Autodesk Fusion 360 part; units mm, degrees
sketch "top view" plane through (0, 0, 0) normal (0, 0, 1) x (1, 0, 0)
  line L0 (12.0004, 0) -> (29.9996, 0)
  line L1 (42, 12) -> (42, 66)
  line L2 (42, 66) -> (0, 66)
  line L3 (0, 66) -> (0, 0) construction
  line L4 (21, 66) -> (21, 0) construction
  line L5 (0, 66) -> (15, 66)
  line L6 (15, 54) -> (15, 0)
  line L7 (15, 0) -> (12.0004, 0) construction
  line L8 (0, 12) -> (0, 66)
  line L9 (27, 54) -> (27, 0)
  line L10 (0, 0) -> (12.0004, 0) construction
  line L11 (12.0004, 0) -> (12.0004, 12) construction
  line L12 (12.0004, 12) -> (0, 12) construction
  line L13 (0, 12) -> (0, 0) construction
  line L14 (0, 12) -> (12.0004, 0)
  line L15 (29.9996, 12) -> (42, 12) construction
  line L16 (29.9996, 0) -> (29.9996, 12) construction
  line L17 (42, 12) -> (29.9996, 0)
  line L18 (42, 12) -> (42, 0) construction
  line L19 (42, 0) -> (29.9996, 0) construction
  line L20 (0, 66) -> (42, 66)
  line L21 (42, 66) -> (42, 54)
  line L22 (42, 54) -> (0, 54)
  line L23 (0, 54) -> (0, 66)
  line L24 (15, 66) -> (15, 54) construction
  line L25 (27, 54) -> (27, 66) construction
  dimension "d1" = 66
  dimension "d3" = 12
  dimension "d4" = 12
extrude "Extrude1" add sketch "top view" along normal blind 12
extrude "Extrude2" add sketch "top view" along normal blind 60 contours L1 L2 L5 L8 L20 L21 L22 L23
fillet "Fillet1" radius 21 2 edges at (0, 60, 60) (42, 60, 60)
extrude "Extrude3" add sketch "top view" along normal blind 54 contours L0 L6 L9 L22
sketch "middle part side view" plane through (0, 0, 0) normal (1, 0, 0) x (0, 1, 0)
  line L0 (0, 12) -> (54, 54)
  line L1 (54, 54) -> (54, 12)
  line L2 (54, 12) -> (0, 12)
  line L3 (0, 54) -> (0, 12)
  line L4 (54, 54) -> (0, 54)
extrude "Extrude4" cut sketch "middle part side view" along normal blind 45 contours L0 L3 L4
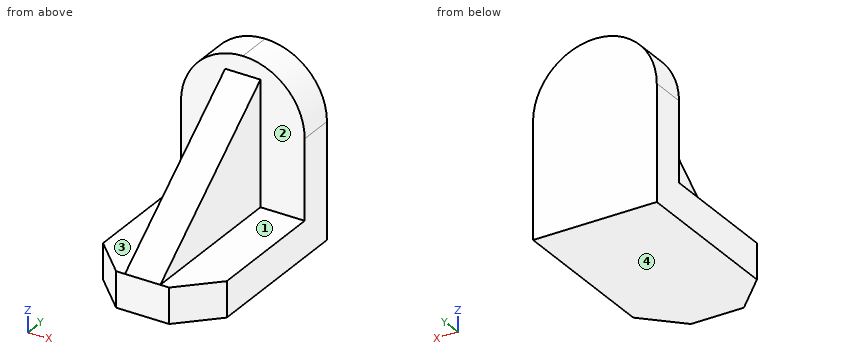
Here's how the part is built. I have some questions about the finished solid (model axes, mm). Face numbers are marked on the shaded views. A direction names the side the tool comes from. Give positions to 0.01 mm unless a question says otherwise; leave off trailing zeros. Order: outer loops, then holes, each group sorted by start corner. A loop starts at its lowest first (then second) coordinate and runs counter-clockwise, first axis right, second up. Notation, with made-up numbers: (-2.5, -3.75) -> (48.5, -3.75) arc R26 cw to (48.5, 35.25) -> close; hole circle Ø2 at (71.5, 44.25). An arc over 180 degrees is marked (long way). Use a Markdown table: item, result. Add a question column.
Item 1: I need wall thicknesses on line 1 (X direction, y = 17, z = 21); line 2 (Z direction, x = 8, y = 29); line 3 (Y direction, x = 30, z = 52). Which ranges of each line are inside material? Lowest first, please.
Item 2: Imagine slicing it at B-B on y = 20.5. Please give me the cut outline in (x, z).
Item 3: Imagine slicing it at C-C on x = 34. Please give me the cut outline in (y, z), plus the area to 3 significant figures.
Item 4: Imagine slicing it at A-A on z = 36.5. Please give me the cut outline in (x, y), plus the area to 3 significant figures.
Item 5: Will these pins go through, and if not, where does the flat tip stop? pin 1 (16.5 mm diameter, centred on x = 36.5, y = 32, fed in from +Z); pin 2 (2 mm diameter, centred on x = 31.5, z = 27, fed in from -Y); pin 3 (10 mm diameter, centred on y = 41.5, z = 29, fed in from +X).
Item 6: For the marked faces 1, 2, 3 and 4, which set-ups out of +Z, -Z, +X, -X, +Y, -Y let a thin tool reach every point of the face, with its end or its side?
Item 7: Imagine slicing it at D-D on z = 11. Please give me the cut outline in (x, y), plus the area to 3 significant figures.
Data:
| question | item | result |
|---|---|---|
| 1 | line 1 | x = 15 to 27 |
| 1 | line 2 | z = 0 to 12 |
| 1 | line 3 | y = 54 to 66 |
| 2 | outline | (0, 0) -> (42, 0) -> (42, 12) -> (27, 12) -> (27, 27.94) -> (15, 27.94) -> (15, 12) -> (0, 12) -> close |
| 3 | outline | (4, 0) -> (66, 0) -> (66, 55.49) -> (54, 55.49) -> (54, 12) -> (4, 12) -> close |
| 3 | area | 1,270 mm² |
| 4 | outline | (0, 54) -> (15, 54) -> (15, 31.5) -> (27, 31.5) -> (27, 54) -> (42, 54) -> (42, 66) -> (0, 66) -> close |
| 4 | area | 774 mm² |
| 5 | pin 1 | stops at z = 12 |
| 5 | pin 2 | stops at y = 54 |
| 5 | pin 3 | stops at x = 27 |
| 6 | face 1 | +Z, +X, -Y |
| 6 | face 2 | +Z, -Y |
| 6 | face 3 | +Z, -X, -Y |
| 6 | face 4 | -Z, +X, -X, +Y, -Y |
| 7 | outline | (0, 12) -> (12, 0) -> (30, 0) -> (42, 12) -> (42, 66) -> (0, 66) -> close |
| 7 | area | 2,630 mm² |
